```python
from build123d import *

# Parameters (mm, degrees)
F1_DEPTH = 12
F2_R     = 5
F3_DEPTH = 9
F5_D     = 6
F7_D     = 6


with BuildPart() as f1:
    # F0 (on Front) → F1 (new body)
    with BuildSketch(Plane.XZ):
        Polygon((3, -11), (6, -11), (6, 11), (-6, 11), (-6, -11), (-3, -11), (-3, 8), (3, 8), align=None)
    extrude(amount=F1_DEPTH)

    # F2 (on face) → F3 (join)
    with BuildSketch(Plane.XY.offset(11)):
        with Locations((0, -6)):
            Circle(F2_R)
    extrude(amount=F3_DEPTH)

    # F5 (through all)
    with Locations(Plane.XY.offset(20)):
        with Locations((0, -6)):
            Hole(F5_D / 2)

    # F7 (through all)
    with Locations(Plane(origin=(-6, 0, 0), x_dir=(0, -1, 0), z_dir=(-1, 0, 0))):
        with Locations((6, -4)):
            Hole(F7_D / 2)


solid = f1.part
```
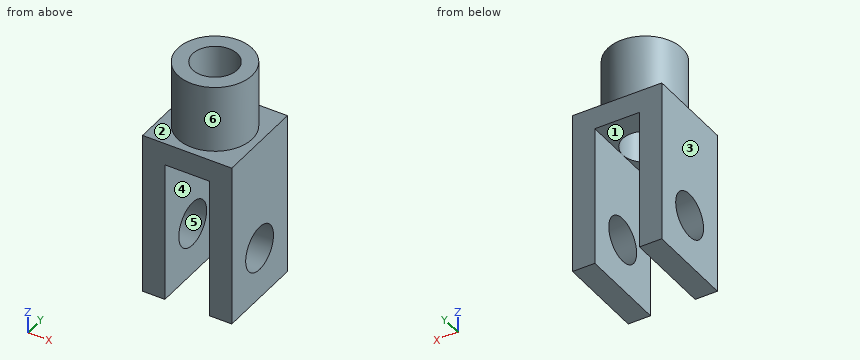
Input: part model. Units: mm. Frame: model coordinates. Face numbers are marked on the shaded views. A direction names the side the tool comes from. Give positions to 0.01 mm unless a question says otherwise; leave off trailing zeros. Order: outer loops, then holes, each group sorted by start corner. A loop starts at its lowest first (then second) coordinate and runs counter-clockwise, first axis right, second up. Notation, with made-up numbers: M 6,68 L 54,68 A9 ccw 54,77 Z; hole C 49,81 d8. An arc over 180 degrees is marked long. One line per question, with ' | ' between items. Start each with the question number.
1. Access query for the marked faces 4, 5 and 6. Directions: +Z, -Z, +X, -X, +Y, -Y. A direction counts if a zero-diameter tool reaches every point of the face in a straight line with its end or side. Return the directions, or none.
2. First-contact query: pin 1 Ø3 at (x, z) = (-3, -1.5) entering from +Y; pin 2 Ø3 at (x, z) = (1.5, 17) entering from -Y. Flat tips, straight axial feed; report the tip coordinate or a pass-through.
3. Section query B-B (z = -4). Return the cut outline in (x, y), and give its area (3 significant figures).
4. Pull-direction query (X, two-part tool) for the marked faces 1, 2 and 3; classes: released by +X, released by -X, zero draft, split by the parting line, or undercut.
5. Material intervals for probe 1 along X at (y, z) = (-5.25, -1); probe 2 along Z at (x, y) = (-5.05, -6); probe 3 along Z at (x, y) = (2.5, -8), sorted ascending. Write a range as [from, to].
6. Section query C-C (x = 0). Return the cut outline in (y, z), and give its area (3 significant figures).
7. Section query D-D (y = -6.5). Return the cut outline in (x, z), and give its area (3 significant figures).
8. Section query A-A (z = 6.5). Return the cut outline in (x, y).
Here are the results:
1) face 4: -Z, +Y, -Y | face 5: +X, -X | face 6: +Z
2) pin 1: y = 0 | pin 2: y = -11
3) outline: M -6,-12 L -3,-12 L -3,-9 L -6,-9 Z; M -6,-3 L -3,-3 L -3,0 L -6,0 Z; M 3,-12 L 6,-12 L 6,-9 L 3,-9 Z; M 3,-3 L 6,-3 L 6,0 L 3,0 Z | area: 36.0 mm²
4) face 1: undercut | face 2: zero draft | face 3: released by -X
5) probe 1: [-6, -3], [3, 6] | probe 2: [-11, -7], [-1, 11] | probe 3: [8, 20]
6) outline: M -12,8 L -9,8 L -9,20 L -11,20 L -11,11 L -12,11 Z; M -3,8 L 0,8 L 0,11 L -1,11 L -1,20 L -3,20 Z | area: 54.0 mm²
7) outline: M -6,-11 L -3,-11 L -3,-6.96 L -6,-6.96 Z; M -6,-1.04 L -3,-1.04 L -3,8 L -2.96,8 L -2.96,20 L -4.97,20 L -4.97,11 L -6,11 Z; M 2.96,8 L 3,8 L 3,-1.04 L 6,-1.04 L 6,11 L 4.97,11 L 4.97,20 L 2.96,20 Z; M 3,-11 L 6,-11 L 6,-6.96 L 3,-6.96 Z | area: 133 mm²
8) outline: M -6,-12 L -3,-12 L -3,0 L -6,0 Z; M 3,-12 L 6,-12 L 6,0 L 3,0 Z
